from build123d import *

# Parameters (mm, degrees)
F0_R     = 37.3207707479
F1_DEPTH = 6
F2_R     = 0.5


# Not quite as in the source:
# - two fillets or chamfers of one size are made in one step


with BuildPart() as f1:
    # F0 (on Front) → F1 (new body)
    with BuildSketch(Plane.XZ):
        Circle(F0_R)
        with BuildLine():
            ThreePointArc((-11.1602745113, -2.7745761537), (-9.9592921435, 5.75), (-3.1772838218, 11.0523693168))
            Line((-3.1772838218, 11.0523693168), (-8, 14.4292715395))
            Line((-8, 14.4292715395), (-8, 25.1894103565))
            ThreePointArc((-8, 25.1894103565), (0, 26.4292715395), (8, 25.1894103565))
            Line((8, 25.1894103565), (8, 14.4292715395))
            Line((8, 14.4292715395), (3.1772838218, 11.0523693168))
            ThreePointArc((3.1772838218, 11.0523693168), (9.9592921435, 5.75), (11.1602745113, -2.7745761537))
            Line((11.1602745113, -2.7745761537), (16.4961157113, -0.2864325395))
            Line((16.4961157113, -0.2864325395), (25.8146692751, -5.666501948))
            ThreePointArc((25.8146692751, -5.666501948), (24.9687771204, -8.6640962149), (23.7761097196, -11.5413604358))
            ThreePointArc((23.7761097196, -11.5413604358), (22.7401432363, -13.4681951166), (21.5483693449, -15.3027504941))
            ThreePointArc((21.5483693449, -15.3027504941), (19.880834384, -17.4143279602), (18.0072512686, -19.3454205397))
            Line((18.0072512686, -19.3454205397), (8.4695163323, -13.8388067068))
            Line((8.4695163323, -13.8388067068), (7.9829906895, -8.2777931631))
            ThreePointArc((7.9829906895, -8.2777931631), (0, -11.5), (-7.9829906895, -8.2777931631))
            Line((-7.9829906895, -8.2777931631), (-8.4961157113, -14.142839))
            Line((-8.4961157113, -14.142839), (-17.8146692751, -19.5229084085))
            ThreePointArc((-17.8146692751, -19.5229084085), (-22.8884205567, -13.2146357697), (-25.8146692751, -5.666501948))
            Line((-25.8146692751, -5.666501948), (-16.4961157113, -0.2864325395))
            Line((-16.4961157113, -0.2864325395), (-11.1602745113, -2.7745761537))
        make_face(mode=Mode.SUBTRACT)
    extrude(amount=F1_DEPTH)

    # F2
    f2_edges = [f1.edges().sort_by_distance(p)[0] for p in [
        (-17.814669, -3, -19.522908),
        (-25.814669, -3, -5.666502),
        (-8.496116, -3, -14.142839),
        (-7.982991, -3, -8.277793),
        (7.982991, -3, -8.277793),
        (8.469516, -3, -13.838807),
        (18.007251, -3, -19.345421),
        (25.814669, -3, -5.666502),
        (16.496116, -3, -0.286433),
        (11.160275, -3, -2.774576),
        (3.177284, -3, 11.052369),
        (8, -3, 14.429272),
        (8, -3, 25.18941),
        (-8, -3, 25.18941),
        (-8, -3, 14.429272),
        (-3.177284, -3, 11.052369),
        (-11.160275, -3, -2.774576),
        (-16.496116, -3, -0.286433),
    ]]
    fillet(f2_edges, radius=F2_R)


solid = f1.part
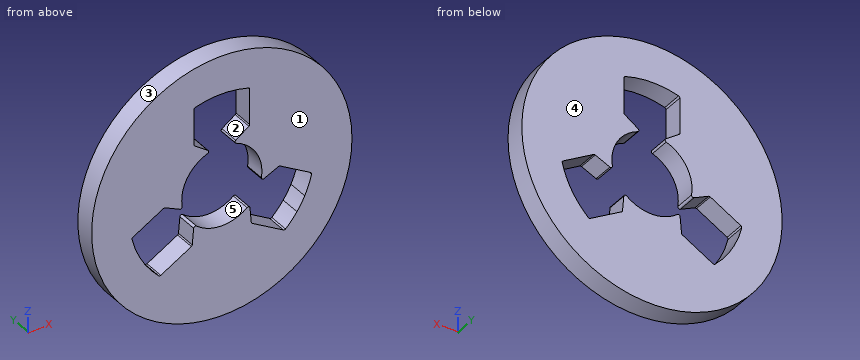
Verification items for the finished model (mm, model axes). Face numbers are marked on the shaded views. A direction names the side the tool comes from. Round coordinates to 2 decimals unless told otherwise and drop trailing zeros. Write each loop counter-clockwise with the first axis right and the second up, starting at its lowest first coordinate (ties: lowest second). Pieces come first, ordered by that corner, then holes.
(1) Mould release check, pull along X, two halves, no side actions. Record for the marked faces 3, 4 and 5: pulls with the +X half, pulls with the -X half, needs draft (parallel to the pull), parting line crosses it, or undercut.
Returned:
face 3: parting line crosses it
face 4: needs draft
face 5: undercut
(2) Material ranges on line 1 (X direction, y = -0.45, z = -15); line 2 (X direction, y = -4.8, z = -1.5); line 3 (Z direction, x = 5, y = -5.45), recorded low to high.
Returned:
line 1: x = -34.17 to -21.76, -9.98 to 10.48, 21.76 to 34.17
line 2: x = -37.29 to -18.6, -13.89 to -11.4, 11.4 to 13.89, 18.6 to 37.29
line 3: z = -36.98 to -10.36, 10.36 to 12.33, 25.95 to 36.98
(3) Section check B-B (z = -7). Enter the section's corners in (x, y), plus the area to 3 significant figures.
Returned:
outline: (-36.66, -6) - (-25.49, -6) - (-25.49, 0) - (-36.66, 0) - close; (25.49, -6) - (36.66, -6) - (36.66, 0) - (25.49, 0) - close
area: 134 mm2
(4) Depth check by flat-ended pin: pin 1 Ø3 at (y, z) = (-2.5, 21) entering from +X; pin 2 Ø1.5 at (y, z) = (-1.5, 5) entering from +X; pin 3 Ø2 at (y, z) = (-4, -21.5) entering from -X. Enter the tip coordinate at first touch or a pass-through.
Returned:
pin 1: stops at x = 31.82
pin 2: stops at x = 37.08
pin 3: stops at x = -31.19
(5) Section check C-C (z = -26). Enter the section's corners in (x, y).
Returned:
outline: (-26.77, -6) - (26.77, -6) - (26.77, 0) - (-26.77, 0) - close
(6) Section check A-A (x = 0). Enter the section's corners in (y, z).
Returned:
outline: (-6, -37.32) - (0, -37.32) - (0, -11.5) - (-6, -11.5) - close; (-6, 26.43) - (0, 26.43) - (0, 37.32) - (-6, 37.32) - close
(7) Section check D-D (x = 27). Enter the section's corners in (y, z), plus the area to 3 significant figures.
Returned:
outline: (-6, -25.77) - (0, -25.77) - (0, 25.77) - (-6, 25.77) - close
area: 309 mm2
(8) Access from +Z, -Z, +X, -X, +Y, -Y to the whole of each face (thin tool, end or side, straight path). Record for the marked faces 1 and 2.
Returned:
face 1: +Z, -Z, +X, -X, -Y
face 2: +Y, -Y
